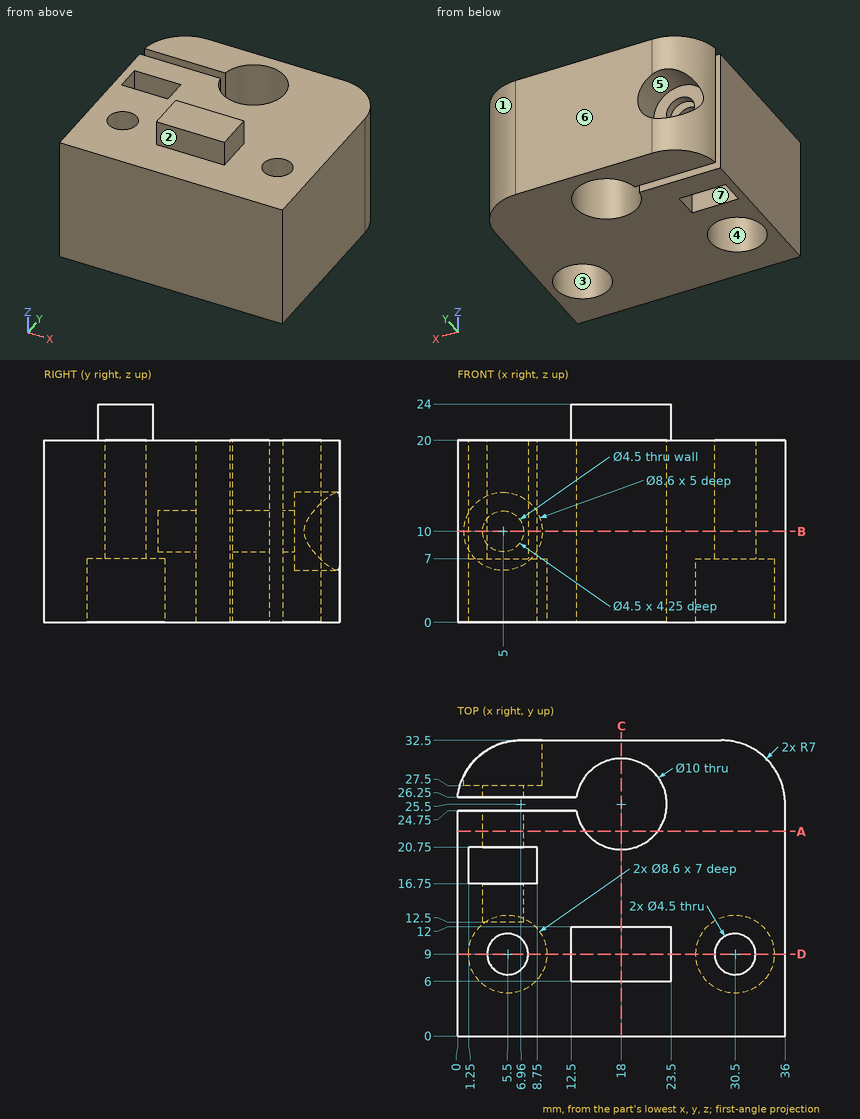
Verification items for this drawing (mm, ordinates from the low corner). A direction names the side the tool comes from. Round coordinates to 2 decimals unless told otherwise and drop trailing zeros. Order: outer loops, then holes, each group sorted by start corner. A loop starts at its lowest first (then second) coordinate and runs counter-clockwise, first axis right, second up.
1) Tool access check on the marked faces 4, 5, 6 and 7. Record the directions out of +Z, -Z, +X, -X, +Y, -Y that give a thin tool (end or side, any length) a straight path to the whole face; none if there is none.
Geometry says:
face 4: -Z
face 5: +Y
face 6: +Z, -Z, +X, -X, +Y
face 7: +Z, -Z
2) Cross-section at A-A, the plane y = 22.5. Record the cut outline in (x, z).
Geometry says:
outline: (0, 0) - (14, 0) - (14, 20) - (0, 20) - close; (22, 0) - (36, 0) - (36, 20) - (22, 20) - close; hole circle Ø4.5 at (5, 10)
3) Depth check by flat-ended pin: pin 1 (7.5 mm diameter, centred on x = 5.5, y = 9, fed in from +Z); pin 2 (7 mm diameter, centred on x = 5, z = 10.5, fed in from +Y); pin 3 (2 mm diameter, centred on y = 8.5, z = 21.5, fed in from +X). Enter the tip coordinate at first touch or a pass-through.
Geometry says:
pin 1: stops at z = 20
pin 2: stops at y = 27.5
pin 3: stops at x = 23.5
4) Cross-section at C-C, the plane x = 18. Record the cut outline in (y, z), plus the area to 3 significant figures.
Geometry says:
outline: (0, 0) - (20.5, 0) - (20.5, 20) - (12, 20) - (12, 24) - (6, 24) - (6, 20) - (0, 20) - close; (30.5, 0) - (32.5, 0) - (32.5, 20) - (30.5, 20) - close
area: 474 mm2
5) Cross-section at B-B, the plane z = 10. Give the number of separate pieces and of enclosed holes in the cut face.
Geometry says:
separate pieces: 2
enclosed holes: 2
6) Draft check along Y on the marked faces 1, 2 and 3. Enter one of: +Y half, -Y half, draft (parallel to the pull), parting line (faces both ways), or undercut.
Geometry says:
face 1: +Y half
face 2: -Y half
face 3: undercut
7) Cross-section at D-D, the plane y = 9. Record the cut outline in (x, z).
Geometry says:
outline: (0, 0) - (1.2, 0) - (1.2, 7) - (3.25, 7) - (3.25, 20) - (0, 20) - close; (7.75, 7) - (9.8, 7) - (9.8, 0) - (26.2, 0) - (26.2, 7) - (28.25, 7) - (28.25, 20) - (23.5, 20) - (23.5, 24) - (12.5, 24) - (12.5, 20) - (7.75, 20) - close; (32.75, 7) - (34.8, 7) - (34.8, 0) - (36, 0) - (36, 20) - (32.75, 20) - close
8) Material ranges on line 1 (Y direction, x = 5.5, z = 13.5); line 2 (Y direction, x = 9.5, z = 9.25); line 3 (Y direction, x = 5.5, z = 15.5), recorded low to high.
Geometry says:
line 1: y = 0 to 6.75, 11.25 to 16.75, 20.75 to 24.75, 26.25 to 27.5
line 2: y = 0 to 24.75, 26.25 to 32.5
line 3: y = 0 to 6.75, 11.25 to 16.75, 20.75 to 24.75, 26.25 to 32.35
